```python
from build123d import *

# Parameters (mm, degrees)
BOSS_EXTRUDE1_DEPTH = 5


with BuildPart() as part:
    # Sketch1 → Boss-Extrude1 (new body)
    with BuildSketch(Plane.XY):
        Polygon((0, 0), (40.395, 0), (40.395, -5), (55.395, -5), (55.395, 0), (65.395, 0), (61.954765166, 7.914471805), (66.540293361, 9.907693111), (62.55385075, 19.078749501), (57.968322555, 17.085528195), (54.528087721, 25), (0, 25), align=None)
    boss_extrude1 = extrude(amount=BOSS_EXTRUDE1_DEPTH)

    # Mirror1: Boss-Extrude1 across plane
    add(boss_extrude1.mirror(Plane(origin=(0, 0, 5), x_dir=(0, 0, 1), z_dir=(1, 0, 0))))


solid = part.part
```
Geometry check sheet. Reference: the model listing, model coordinates, mm. A direction names the side the tool comes from. Round coordinates to 2 decimals unless told otherwise and drop trailing zeros. Loops run counter-clockwise (first coordinate to the right, second up) from the corner with the lowest first, then second, coordinate; pieces in that order, holes last. Notation, with made-up numbers: M 40.25,37 L 51.25,37 A5 ccw 51.25,46 Z; hole C -3.75,-35.5 d11. An arc over 180 degrees is marked long. Return JSON: item names as keys, results as strings. Group by question number.
(1) Section check D-D, the plane y = 20.25. Enter the section's corners in (x, z), and give its area (3 significant figures).
(2) Scan lines: line 1 along X through (y, z) = (-0.75, 1.6) (3 decimals); line 2 along X through (y, z) = (17.25, 1.5); line 3 along Y through (x, z) = (13, 3.1). Record each from-to range of solid material in increasing order. Write a range as [from, to].
(3) Set-up check for faces 1 (the face through (-60, 0, 2)), 2 (the face through (63.7, 3.9, 2.5)), 3 (the face through (-64.22, 8.9, 2.46)), 4 (the face through (-56.27, 20.99, 2.46)): record each of +Z, -Z, +X, -X, +Y, -Y from which the full face is reachable in a straight line by a thin tool's end or side.
(4) Mould release check, pull along X, two halves, no side actions. Record for faces 5 (the face through (-60.3, 18.1, 2.5)), 6 (the face through (55.395, -3, 2)), 7 (the face through (48, -5, 2)): pulls with the +X half, pulls with the -X half, needs draft (parallel to the pull), parting line crosses it, or undercut.
(5) Go/stop test with flat-tipped pins: pin 1 (1.5 mm diameter, centred on y = -2.5, z = 3, fed in from +X) (3 decimals); pin 2 (1.5 mm diameter, centred on x = -58, z = 3.5, fed in from -Y); pin 3 (1.5 mm diameter, centred on y = -1.5, z = 3.5, fed in from -X) (3 decimals). Record where each tip stops, or that it passes through.
(6) Section check A-A, the plane y = -2.25. Enter the section's corners in (x, z) (3 decimals), and give its area (3 significant figures).
(7) Section check B-B, the plane z = 3.6. Enter the section's corners in (x, y) (3 decimals).
(8) Section check C-C, the plane x = -7. Enter the section's corners in (y, z), and give its area (3 significant figures).
Data:
{
 "1": {"outline": "M -56.59,0 L 56.59,0 L 56.59,5 L -56.59,5 Z", "area": "566 mm²"},
 "2": {"line 1": "[-55.395, -40.395], [40.395, 55.395]", "line 2": "[-63.35, -58.35], [-57.9, 57.9], [58.35, 63.35]", "line 3": "[0, 25]"},
 "3": {"face 1": "+Z, -Z, -X, -Y", "face 2": "+Z, -Z, +X", "face 3": "+Z, -Z, -X", "face 4": "+Z, -Z, +Y"},
 "4": {"face 5": "undercut", "face 6": "pulls with the +X half", "face 7": "needs draft"},
 "5": {"pin 1": "x = 55.395", "pin 2": "y = 0", "pin 3": "x = -55.395"},
 "6": {"outline": "M -55.395,0 L -40.395,0 L -40.395,5 L -55.395,5 Z; M 40.395,0 L 55.395,0 L 55.395,5 L 40.395,5 Z", "area": "150 mm²"},
 "7": {"outline": "M -66.54,9.908 L -61.955,7.914 L -65.395,0 L -55.395,0 L -55.395,-5 L -40.395,-5 L -40.395,0 L 40.395,0 L 40.395,-5 L 55.395,-5 L 55.395,0 L 65.395,0 L 61.955,7.914 L 66.54,9.908 L 62.554,19.079 L 57.968,17.086 L 54.528,25 L -54.528,25 L -57.968,17.086 L -62.554,19.079 Z"},
 "8": {"outline": "M 0,0 L 25,0 L 25,5 L 0,5 Z", "area": "125 mm²"}
}
